from build123d import *

# Parameters (mm, degrees)
ESQUISSE1_R        = 1
BOSS_EXTRU_1_DEPTH = 6


with BuildPart() as part:
    # Esquisse1 → Boss.-Extru.1 (new body)
    with BuildSketch(Plane.XY):
        with BuildLine():
            Line((-5.125601059, 7.752865214), (-7.025601059, 7.294584696))
            ThreePointArc((-7.025601059, 7.294584696), (-7.501583822, 7.432360963), (-7.625219148, 7.912211144))
            Line((-7.625219148, 7.912211144), (-8.091799231, 10.912211144))
            ThreePointArc((-8.091799231, 10.912211144), (-7.52044361, 12.313188257), (-6.015074536, 12.46500415))
            Line((-6.015074536, 12.46500415), (-3.79657697, 11.417824019))
            ThreePointArc((-3.79657697, 11.417824019), (-3.501096688, 11.418143301), (-3.314034571, 11.646871225))
            Line((-3.314034571, 11.646871225), (-5.170456982, 13.403293241))
            ThreePointArc((-5.170456982, 13.403293241), (-5.667222651, 13.720510456), (-6.246087907, 13.831496523))
            ThreePointArc((-6.246087907, 13.831496523), (-7.702827431, 13.804605734), (-9.157582062, 13.723970009))
            ThreePointArc((-9.157582062, 13.723970009), (-10.266440997, 13.409307705), (-11.057492389, 12.570965175))
            Line((-11.057492389, 12.570965175), (-16.083035607, -1.602809651))
            Line((-16.083035607, -1.602809651), (-16.083035607, -23.988240086))
            ThreePointArc((-16.083035607, -23.988240086), (-15.599388885, -25.155866561), (-14.43176241, -25.639513283))
            Line((-14.43176241, -25.639513283), (-13.486808234, -25.97456221))
            Line((-13.486808234, -25.97456221), (-10.920669924, -25.35560895))
            Line((-10.920669924, -25.35560895), (-10.920669924, -24.556164823))
            Line((-10.920669924, -24.556164823), (-13.486808234, -23.646298599))
            Line((-13.486808234, -23.646298599), (-13.486808234, -3.776370077))
            Line((-13.486808234, -3.776370077), (-11.927338138, 0.621876447))
            ThreePointArc((-11.927338138, 0.621876447), (-11.717055765, 1.352491988), (-11.057492389, 1.73063733))
            Line((-11.057492389, 1.73063733), (-4.515694846, 2.623090489))
            ThreePointArc((-4.515694846, 2.623090489), (-1.932742353, 5.531336315), (-5.125601059, 7.752865214))
        make_face()
        with Locations((-4.515694846, 5.224235349)):
            Circle(ESQUISSE1_R, mode=Mode.SUBTRACT)
    extrude(amount=BOSS_EXTRU_1_DEPTH)


solid = part.part
Check sheet for the modelled part. Datum: model origin and axes. Units: mm. A direction names the side the tool comes from. Round coordinates to 2 decimals unless told otherwise and drop trailing zeros. Loops run counter-clockwise (first coordinate to the right, second up) from the corner with the lowest first, then second, coordinate; pieces in that order, holes last.
1. Gauge pin test, flat ends, axial feed: pin 1 Ø1 at (y, z) = (-13, 2) entering from +X; pin 2 Ø3 at (y, z) = (-5, 3.5) entering from +X; pin 3 Ø1.6 at (x, y) = (-4.52, 5.22) entering from +Z; pin 4 Ø2 at (x, z) = (-6, 5) entering from -Y. Record the tip position at first contact, or that the pin passes through.
2. Scan lines: probe 1 along Y at (x, z) = (-4.75, 2.85); probe 2 along Y at (x, z) = (-5, 1.15); probe 3 along X at (y, z) = (-6.5, 5.2). Record each from-to range of solid material in increasing order.
3. Sectioned sample at C-C on y = -6. Record the boundary of the cut face in (x, z).
4. Sectioned sample at A-A on x = -11.5. Record the boundary of the cut face in (y, z).
5. Mould release check, pull along X, two halves, no side actions. Record for faces 1 (the cylindrical face through (-10.25, 13.42, 2.96)), 2 (the flat face through (-12.22, -25.67, 2.96)), 3 (the flat face through (-4.92, 11.95, 2.96)): released by +X, released by -X, zero draft, split by the parting line, or undercut.
6. Set-up check for faces 4 (the flat face through (-4.229, 12.513, 2.958)), 5 (the flat face through (-7.855, 9.391, 2.958)): record each of +Z, -Z, +X, -X, +Y, -Y from which the full face is reachable in a straight line by a thin tool's end or side.
7. Sectioned sample at D-D on x = -9.5. Record the boundary of the cut face in (y, z).
8. Sectioned sample at B-B on z = 1.5. Record the boundary of the cut face in (x, y) (1 decimal), and give its area (3 significant figures).
Recorded:
1. pin 1: stops at x = -13.49
1. pin 2: stops at x = -13.39
1. pin 3: passes through
1. pin 4: stops at y = 2.28
2. probe 1: y = 2.59 to 4.25, 6.2 to 7.81, 11.87 to 13.01
2. probe 2: y = 2.56 to 4.35, 6.1 to 7.78, 11.99 to 13.24
2. probe 3: x = -16.08 to -13.49
3. outline: (-16.08, 0) - (-13.49, 0) - (-13.49, 6) - (-16.08, 6) - close
4. outline: (-25.5, 0) - (-24.35, 0) - (-24.35, 6) - (-25.5, 6) - close; (1.56, 0) - (11.32, 0) - (11.32, 6) - (1.56, 6) - close
5. face 1: released by -X
5. face 2: released by +X
5. face 3: undercut
6. face 4: +Z, -Z, +X, +Y
6. face 5: +Z, -Z, +X
7. outline: (1.94, 0) - (13.69, 0) - (13.69, 6) - (1.94, 6) - close
8. outline: (-16.1, -24) arc R1.7 ccw to (-14.4, -25.6) - (-13.5, -26) - (-10.9, -25.4) - (-10.9, -24.6) - (-13.5, -23.6) - (-13.5, -3.8) - (-11.9, 0.6) arc R1 cw to (-11.1, 1.7) - (-4.5, 2.6) arc R2.6 ccw (long way) to (-5.1, 7.8) - (-7, 7.3) arc R0.5 cw to (-7.6, 7.9) - (-8.1, 10.9) arc R1.5 cw to (-6, 12.5) - (-3.8, 11.4) arc R0.3 ccw to (-3.3, 11.6) - (-5.2, 13.4) arc R1.6 ccw to (-6.2, 13.8) arc R39.5 ccw to (-9.2, 13.7) arc R2.2 ccw to (-11.1, 12.6) - (-16.1, -1.6) - close; hole circle Ø2 at (-4.5, 5.2)
8. area: 166 mm2
